Geometry check sheet. Reference: the model listing, model coordinates, mm. A direction names the side the tool comes from. Coordinates: 2 decimals unless noted, no trailing zeros. Write each loop counter-clockwise with the first axis right and the second up, starting at its lowest first coordinate (ties: lowest second). Pieces come first, ordered by that corner, then holes. Notation, with made-up numbers: M -16.5,-11 L 13.5,-11 A28 ccw 13.5,16 Z; hole C -32.75,-30 d10. An arc over 180 degrees is marked long. Write each question's results on one line, items separated by ' | '.
```python
from build123d import *

# Parameters (mm, degrees)
F1_W     = 1219.2
F1_H     = 1600.2
F2_DEPTH = 50.8
F3_R     = 57.15
F4_DEPTH = 76.2
F5_W     = 304.8
F5_H     = 101.6
F5_H_2   = 152.4
F6_DEPTH = 76.2
F7_DEPTH = 76.2


with BuildPart() as f2:
    # F1 (on face) → F2 (new body)
    with BuildSketch(Plane.XZ):
        Rectangle(F1_W, F1_H)
    extrude(amount=F2_DEPTH)

    # F3 (on face) → F4 (cut)
    with BuildSketch(Plane.XZ.offset(50.8)):
        with Locations((-482.6, 673.1)):
            Circle(F3_R)
        with Locations((482.6, 673.1)):
            Circle(F3_R)
        with Locations((-482.6, -673.1)):
            Circle(F3_R)
        with Locations((482.6, -673.1)):
            Circle(F3_R)
    extrude(amount=-F4_DEPTH, mode=Mode.SUBTRACT)

    # F5 (on face) → F6 (cut)
    with BuildSketch(Plane.XZ.offset(50.8)):
        with Locations((0, 177.8)):
            Rectangle(F5_W, F5_H)
        with BuildLine():
            ThreePointArc((-152.4, 228.6), (-203.2, 177.8), (-152.4, 127))
            Line((-152.4, 127), (-152.4, 228.6))
        make_face()
        with BuildLine():
            Line((152.4, 228.6), (152.4, 127))
            ThreePointArc((152.4, 127), (203.2, 177.8), (152.4, 228.6))
        make_face()
        with BuildLine():
            Line((152.4, -127), (-152.4, -127))
            ThreePointArc((-152.4, -127), (-203.2, -177.8), (-152.4, -228.6))
            Line((-152.4, -228.6), (152.4, -228.6))
            ThreePointArc((152.4, -228.6), (203.2, -177.8), (152.4, -127))
        make_face()
        Rectangle(F5_W, F5_H_2)
        with BuildLine():
            ThreePointArc((-152.4, 76.2), (-228.6, 0), (-152.4, -76.2))
            Line((-152.4, -76.2), (-152.4, 76.2))
        make_face()
        with BuildLine():
            Line((152.4, 76.2), (152.4, -76.2))
            ThreePointArc((152.4, -76.2), (228.6, 0), (152.4, 76.2))
        make_face()
    extrude(amount=-F6_DEPTH, mode=Mode.SUBTRACT)

    # F5 (on face) → F7 (cut)
    with BuildSketch(Plane.XZ.offset(50.8)):
        with Locations((0, 177.8)):
            Rectangle(F5_W, F5_H)
        with BuildLine():
            ThreePointArc((-152.4, 228.6), (-203.2, 177.8), (-152.4, 127))
            Line((-152.4, 127), (-152.4, 228.6))
        make_face()
        with BuildLine():
            Line((152.4, 228.6), (152.4, 127))
            ThreePointArc((152.4, 127), (203.2, 177.8), (152.4, 228.6))
        make_face()
        with BuildLine():
            Line((152.4, -127), (-152.4, -127))
            ThreePointArc((-152.4, -127), (-203.2, -177.8), (-152.4, -228.6))
            Line((-152.4, -228.6), (152.4, -228.6))
            ThreePointArc((152.4, -228.6), (203.2, -177.8), (152.4, -127))
        make_face()
        Rectangle(F5_W, F5_H_2)
        with BuildLine():
            ThreePointArc((-152.4, 76.2), (-228.6, 0), (-152.4, -76.2))
            Line((-152.4, -76.2), (-152.4, 76.2))
        make_face()
        with BuildLine():
            Line((152.4, 76.2), (152.4, -76.2))
            ThreePointArc((152.4, -76.2), (228.6, 0), (152.4, 76.2))
        make_face()
    extrude(amount=-F7_DEPTH, mode=Mode.SUBTRACT)


solid = f2.part
```
Q1. Mould release check, pull along X, two halves, no side actions. Record for faces 3 (the flat face through (609.6, -25, -11)), 4 (the flat face through (262, 0, 11)), 5 (the cylindrical face through (203.188, -25.756, -178.917)): pulls with the +X half, pulls with the -X half, needs draft (parallel to the pull), parting line crosses it, or undercut.
Geometry check:
face 3: pulls with the +X half | face 4: needs draft | face 5: undercut
Q2. Sectioned sample at C-C on y = -12. Record the cut outline in (x, z), and give its area (3 significant figures).
Geometry check:
outline: M -609.6,-800.1 L 609.6,-800.1 L 609.6,800.1 L -609.6,800.1 Z; hole C -482.6,-673.1 d114.3; hole C -482.6,673.1 d114.3; hole M -152.4,-228.6 L 152.4,-228.6 A50.8 ccw 152.4,-127 L -152.4,-127 A50.8 ccw Z; hole M -152.4,-76.2 L 152.4,-76.2 A76.2 ccw 152.4,76.2 L -152.4,76.2 A76.2 ccw Z; hole M -152.4,127 L 152.4,127 A50.8 ccw 152.4,228.6 L -152.4,228.6 A50.8 ccw Z; hole C 482.6,-673.1 d114.3; hole C 482.6,673.1 d114.3 | area: 1,770,000 mm2
Q3. Sectioned sample at D-D on z = 673.1. Record the cut outline in (x, y).
Geometry check:
outline: M -609.6,-50.8 L -539.75,-50.8 L -539.75,0 L -609.6,0 Z; M -425.45,-50.8 L 425.45,-50.8 L 425.45,0 L -425.45,0 Z; M 539.75,-50.8 L 609.6,-50.8 L 609.6,0 L 539.75,0 Z
Q4. Sectioned sample at B-B on x = -482.6. Record the cut outline in (y, z), and give its area (3 significant figures).
Geometry check:
outline: M -50.8,-800.1 L 0,-800.1 L 0,-730.25 L -50.8,-730.25 Z; M -50.8,-615.95 L 0,-615.95 L 0,615.95 L -50.8,615.95 Z; M -50.8,730.25 L 0,730.25 L 0,800.1 L -50.8,800.1 Z | area: 69,700 mm2
Q5. Sectioned sample at A-A on z = 0. Record the cut outline in (x, y).
Geometry check:
outline: M -609.6,-50.8 L -228.6,-50.8 L -228.6,0 L -609.6,0 Z; M 228.6,-50.8 L 609.6,-50.8 L 609.6,0 L 228.6,0 Z
Q6. Scan lines: probe 1 along Z at (x, y) = (482, -39); probe 2 along X at (y, z) = (-21, -673); probe 3 along Z at (x, y) = (-507.5, -44). Record each from-to range of solid material in increasing order.
Geometry check:
probe 1: z = -800.1 to -730.25, -615.95 to 615.95, 730.25 to 800.1 | probe 2: x = -609.6 to -539.75, -425.45 to 425.45, 539.75 to 609.6 | probe 3: z = -800.1 to -724.54, -621.66 to 621.66, 724.54 to 800.1
Q7. Access from +Z, -Z, +X, -X, +Y, -Y to the whole of each face (thin tool, end or side, straight path). Record for faces 1 (the flat face through (-9, -25, -800.1)), 2 (the flat face through (-2, -26, 228.6)).
Geometry check:
face 1: -Z, +X, -X, +Y, -Y | face 2: +Y, -Y
